Read the model definition and answer for the solid it produces. Units are mm, in the model's axes. Face numbers are marked on the shaded views. A direction names the side the tool comes from. Give positions to 0.01 mm unless a question says otherwise; leave off trailing zeros. Loops run counter-clockwise (first coordinate to the right, second up) from the corner with the lowest first, then second, coordinate; pieces in that order, holes last. Notation, with made-up numbers: (71, 41) - (100, 41) arc R31 ccw to (100, 71) - close; hole circle Ø8 at (30, -32.75). An arc over 180 degrees is marked (long way). Use a Markdown table: item, result. Add a question column.
Item 1: For a pull along X with two mould halves and no side action, classify the marked faces 3, 4 and 5 as +X half, -X half, draft (parallel to the pull), parting line (faces both ways), or undercut.
Item 2: Which of the six approach directions +Z, -Z, +X, -X, +Y, -Y give full straight-line access (tool end or side, diameter ignored) to the marked faces 1 and 2?
Item 3: Consider probe 1 along Z at (x, y) = (7, 1.5); probe 2 along X at (y, z) = (2.25, -5.5); probe 3 along X at (y, z) = (-5.5, -4.25). Determine where each line is inside the solid, lowest interval first. Write a range as [from, to].
Item 4: A cutting plane is placed at D-D (y = 2). Determine the outline of the cut face in (x, z), plus the area to 3 significant figures.
Item 5: A cutting plane is placed at A-A (y = 9). Determine the outline of the cut face in (x, z).
Item 6: A cutting plane is placed at B-B (z = -5.5). Determine the outline of the cut face in (x, y).
Item 7: Each of these flat-tipped pins is pushed along its axis until it touches: P1, Ø4, axis at x = -6, z = -2, coming from the -Y side; P2, Ø1.5, axis at x = 3, y = 5.5, coming from the +Z side; P3, Ø4, axis at y = -10, z = -2.5, coming from the -X side. Where does it stop, or does it pass through?
Item 8: A cutting plane is placed at C-C (y = -4.5). Determine the outline of the cut face in (x, z), plus the area to 3 significant figures.
from build123d import *

# Parameters (mm, degrees)
SKETCH_1_R               = 15
DIAMETER30_HEIGHT8_DEPTH = 8
CHARACTER_DEPTH          = 0.1
SKETCH_3_R               = 13.1
SKETCH_3_R_2             = 12.7
INK_RING_DEPTH           = 0.08


with BuildPart() as part:
    # 草图1 → Diameter30_Height8 (new body)
    with BuildSketch(Plane.XY):
        Circle(SKETCH_1_R)
    extrude(amount=-DIAMETER30_HEIGHT8_DEPTH)

    # 草图2 → Character_士 (add)
    with BuildSketch(Plane.XY):
        with BuildLine():
            add(Edge.make_bspline(
                [(0.824561404, 6.026315789), (0.813336636, 5.83662132), (0.790538423, 5.45133988), (0.771428603, 4.863755794), (0.757740418, 4.258132362), (0.755515021, 3.84828648), (0.754385965, 3.640350877)],
                knots=[0, 0, 0, 0, 0.955126267, 1.939921735, 2.954817811, 4, 4, 4, 4], degree=3))
            Line((0.754385965, 3.640350877), (0.754385965, -0.00877193))
            Line((0.754385965, -0.00877193), (4.964912281, -0.00877193))
            add(Edge.make_bspline(
                [(4.964912281, -0.00877193), (5.184108112, -0.007529011), (5.640726, -0.004939824), (6.351162704, 0.009012072), (7.114519154, 0.028890494), (7.640265954, 0.050317465), (7.912280702, 0.061403509)],
                knots=[0, 0, 0, 0, 0.89213577, 1.858452998, 2.891990654, 4, 4, 4, 4], degree=3))
            Line((7.912280702, 0.061403509), (7.912280702, -1.412280702))
            add(Edge.make_bspline(
                [(7.912280702, -1.412280702), (7.427185378, -1.392141242), (6.468519002, -1.352340771), (5.509053521, -1.345489646), (5.035087719, -1.342105263)],
                knots=[0, 0, 0, 0, 1.012021148, 2, 2, 2, 2], degree=3))
            Line((5.035087719, -1.342105263), (0.754385965, -1.342105263))
            Line((0.754385965, -1.342105263), (0.754385965, -8.219298246))
            Line((0.754385965, -8.219298246), (3.631578947, -8.219298246))
            add(Edge.make_bspline(
                [(3.631578947, -8.219298246), (3.848176317, -8.218087826), (4.292668001, -8.215603856), (4.977115293, -8.20161515), (5.696306453, -8.181989949), (6.187377565, -8.160246287), (6.438596491, -8.149122807)],
                knots=[0, 0, 0, 0, 0.925596292, 1.899468382, 2.925423867, 4, 4, 4, 4], degree=3))
            Line((6.438596491, -8.149122807), (6.438596491, -9.622807018))
            add(Edge.make_bspline(
                [(6.438596491, -9.622807018), (6.22377323, -9.611572963), (5.785618359, -9.588659914), (5.114015233, -9.569582266), (4.416560018, -9.555980066), (3.942610691, -9.553759864), (3.701754386, -9.552631579)],
                knots=[0, 0, 0, 0, 0.942753637, 1.922846234, 2.944411245, 4, 4, 4, 4], degree=3))
            Line((3.701754386, -9.552631579), (-3.666666667, -9.552631579))
            add(Edge.make_bspline(
                [(-3.666666667, -9.552631579), (-3.919651707, -9.553757661), (-4.416990585, -9.555971406), (-5.149099093, -9.569586009), (-5.855343836, -9.588750323), (-6.316905199, -9.61158096), (-6.543859649, -9.622807018)],
                knots=[0, 0, 0, 0, 1.05470571, 2.07342756, 3.052684594, 4, 4, 4, 4], degree=3))
            Line((-6.543859649, -9.622807018), (-6.543859649, -8.149122807))
            add(Edge.make_bspline(
                [(-6.543859649, -8.149122807), (-6.326438065, -8.160395624), (-5.876165846, -8.183741218), (-5.178554503, -8.202420094), (-4.436918096, -8.216076814), (-3.928315814, -8.218203947), (-3.666666667, -8.219298246)],
                knots=[0, 0, 0, 0, 0.907617697, 1.879643343, 2.909187922, 4, 4, 4, 4], degree=3))
            Line((-3.666666667, -8.219298246), (-0.789473684, -8.219298246))
            Line((-0.789473684, -8.219298246), (-0.789473684, -1.342105263))
            Line((-0.789473684, -1.342105263), (-5.140350877, -1.342105263))
            add(Edge.make_bspline(
                [(-5.140350877, -1.342105263), (-5.390737734, -1.343192376), (-5.875950755, -1.345299041), (-6.582068481, -1.358952048), (-7.244168345, -1.377670192), (-7.671036038, -1.401009107), (-7.877192982, -1.412280702)],
                knots=[0, 0, 0, 0, 1.097340975, 2.126485934, 3.095181147, 4, 4, 4, 4], degree=3))
            Line((-7.877192982, -1.412280702), (-7.877192982, 0.061403509))
            add(Edge.make_bspline(
                [(-7.877192982, 0.061403509), (-7.671036038, 0.050131914), (-7.244168345, 0.026792999), (-6.582068481, 0.008074855), (-5.875950755, -0.005578152), (-5.390737734, -0.007684817), (-5.140350877, -0.00877193)],
                knots=[0, 0, 0, 0, 0.904818853, 1.873514066, 2.902659025, 4, 4, 4, 4], degree=3))
            Line((-5.140350877, -0.00877193), (-0.789473684, -0.00877193))
            Line((-0.789473684, -0.00877193), (-0.789473684, 3.640350877))
            add(Edge.make_bspline(
                [(-0.789473684, 3.640350877), (-0.790602741, 3.84828648), (-0.792828137, 4.258132362), (-0.806516322, 4.863755794), (-0.825626143, 5.45133988), (-0.848424355, 5.83662132), (-0.859649123, 6.026315789)],
                knots=[0, 0, 0, 0, 1.045182189, 2.060078265, 3.044873733, 4, 4, 4, 4], degree=3))
            Line((-0.859649123, 6.026315789), (0.824561404, 6.026315789))
        make_face()
    extrude(amount=CHARACTER_DEPTH)

    # 草图3 → Ink_ring (add)
    with BuildSketch(Plane.XY):
        with Locations(Location((0, 0, 0), (0, 0, 180))):
            Circle(SKETCH_3_R)
        with Locations(Location((0, 0, 0), (0, 0, 180))):
            Circle(SKETCH_3_R_2, mode=Mode.SUBTRACT)
    extrude(amount=INK_RING_DEPTH)


solid = part.part
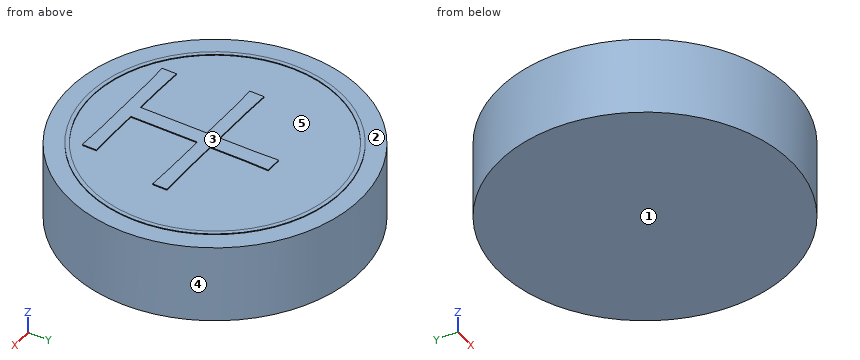
Geometry says:
| question | item | result |
|---|---|---|
| 1 | face 3 | draft |
| 1 | face 4 | parting line |
| 1 | face 5 | undercut |
| 2 | face 1 | -Z, +X, -X, +Y, -Y |
| 2 | face 2 | +Z |
| 3 | probe 1 | [-8, 0] |
| 3 | probe 2 | [-14.83, 14.83] |
| 3 | probe 3 | [-13.96, 13.96] |
| 4 | outline | (-14.87, -8) - (14.87, -8) - (14.87, 0) - (12.95, 0) - (12.95, 0.08) - (12.54, 0.08) - (12.54, 0) - (0.75, 0) - (0.75, 0.1) - (-0.79, 0.1) - (-0.79, 0) - (-12.54, 0) - (-12.54, 0.08) - (-12.95, 0.08) - (-12.95, 0) - (-14.87, 0) - close |
| 4 | area | 238 mm² |
| 5 | outline | (-12, -8) - (12, -8) - (12, 0) - (9.52, 0) - (9.52, 0.08) - (8.96, 0.08) - (8.96, 0) - (-8.96, 0) - (-8.96, 0.08) - (-9.52, 0.08) - (-9.52, 0) - (-12, 0) - close |
| 6 | outline | circle Ø30 at (0, 0) |
| 7 | P1 | y = -14.46 |
| 7 | P2 | z = 0 |
| 7 | P3 | x = -12.69 |
| 8 | outline | (-14.31, -8) - (14.31, -8) - (14.31, 0) - (12.3, 0) - (12.3, 0.08) - (11.88, 0.08) - (11.88, 0) - (0.75, 0) - (0.75, 0.1) - (-0.79, 0.1) - (-0.79, 0) - (-11.88, 0) - (-11.88, 0.08) - (-12.3, 0.08) - (-12.3, 0) - (-14.31, 0) - close |
| 8 | area | 229 mm² |
